Check sheet for the modelled part. Datum: model origin and axes. Units: mm. Face numbers are marked on the shaded views. A direction names the side the tool comes from. Round coordinates to 2 decimals unless told otherwise and drop trailing zeros. Loops run counter-clockwise (first coordinate to the right, second up) from the corner with the lowest first, then second, coordinate; pieces in that order, holes last. Notation, with made-up numbers: M -2,44.25 L 29,44.25 A12 ccw 29,55.25 Z; hole C -24.75,75 d2. An arc over 180 degrees is marked long. Write item = value, one per line. Start each with the question number.
(1) Set-up check for the marked faces 1 and 2: record each of +Z, -Z, +X, -X, +Y, -Y from which the full face is reachable in a straight line by a thin tool's end or side.
(2) Scan lines: L1, parallel to X at y = -7.25, z = 10.5; L2, parallel to X at y = -2.25, z = 14; L3, parallel to X at y = -1.5, z = -3.75. Record each from-to range of solid material in increasing order. Write a range as from..to.
(3) Cross-section at A-A on z = 2.75. Record the boundary of the cut face in (x, y), plus the area to 3 significant figures.
(4) Mould release check, pull along X, two halves, no side actions. Record for the marked faces 3, 4 and 5: pulls with the +X half, pulls with the -X half, needs draft (parallel to the pull), parting line crosses it, or undercut.
(5) Cross-section at C-C on y = -4.5. Record the boundary of the cut face in (x, z), plus the area to 3 significant figures.
(6) Cross-section at B-B on x = -12.5. Record the boundary of the cut face in (y, z).
(7) Cross-section at D-D on z = 11.5. Record the boundary of the cut face in (x, y), plus the area to 3 significant figures.
(8) Go/stop test with flat-tipped pins: P1, Ø2, axis at y = -10, z = 12, coming from the -X side; P2, Ø3, axis at y = -16, z = -1, coming from the +X side; P3, Ø1.5, axis at y = -8.5, z = 15, coming from the -X side. Record where each tip stops, or that it passes through.
from build123d import *

# Parameters (mm, degrees)
F0_R     = 1.5
F0_R_2   = 8.35
F1_DEPTH = 3
F2_DEPTH = 18
F3_R     = 3


with BuildPart() as f1:
    # F0 (on Front) → F1 (new body)
    with BuildSketch(Plane.XZ):
        Polygon((-48.303484, 19.342105), (-48.303484, 8.342105), (-37.303484, 19.342105), align=None)
        with Locations((-45.303484, 16.342105)):
            Circle(F0_R, mode=Mode.SUBTRACT)
        Polygon((-48.303484, 5.342105), (-48.303484, -5.657895), (-37.303484, -5.657895), align=None)
        with Locations((-45.303484, -2.657895)):
            Circle(F0_R, mode=Mode.SUBTRACT)
        Polygon((-48.303484, 5.342105), (-37.303484, -5.657895), (45.696516, -5.657895), (56.696516, 5.342105), (56.696516, 6.842105), (56.696516, 8.342105), (45.696516, 19.342105), (-37.303484, 19.342105), (-48.303484, 8.342105), (-48.303484, 6.842105), align=None)
        with Locations((-33.303484, 6.842105)):
            Circle(F0_R_2, mode=Mode.SUBTRACT)
        with Locations((-8.303484, 6.842105)):
            Circle(F0_R_2, mode=Mode.SUBTRACT)
        with Locations((16.696516, 6.842105)):
            Circle(F0_R_2, mode=Mode.SUBTRACT)
        with Locations((41.696516, 6.842105)):
            Circle(F0_R_2, mode=Mode.SUBTRACT)
        Polygon((45.696516, 19.342105), (56.696516, 8.342105), (56.696516, 19.342105), align=None)
        with Locations((53.696516, 16.342105)):
            Circle(F0_R, mode=Mode.SUBTRACT)
        Polygon((56.696516, 5.342105), (45.696516, -5.657895), (56.696516, -5.657895), align=None)
        with Locations((53.696516, -2.657895)):
            Circle(F0_R, mode=Mode.SUBTRACT)
    extrude(amount=F1_DEPTH)

    # F0 (on Front) → F2 (join)
    with BuildSketch(Plane.XZ):
        Polygon((-48.303484, 5.342105), (-37.303484, -5.657895), (45.696516, -5.657895), (56.696516, 5.342105), (56.696516, 6.842105), (56.696516, 8.342105), (45.696516, 19.342105), (-37.303484, 19.342105), (-48.303484, 8.342105), (-48.303484, 6.842105), align=None)
        with Locations((-33.303484, 6.842105)):
            Circle(F0_R_2, mode=Mode.SUBTRACT)
        with Locations((-8.303484, 6.842105)):
            Circle(F0_R_2, mode=Mode.SUBTRACT)
        with Locations((16.696516, 6.842105)):
            Circle(F0_R_2, mode=Mode.SUBTRACT)
        with Locations((41.696516, 6.842105)):
            Circle(F0_R_2, mode=Mode.SUBTRACT)
    extrude(amount=F2_DEPTH)

    # F3
    f3_edges = [f1.edges().sort_by_distance(p)[0] for p in [
        (-48.303484, -10.5, 8.342105),
        (-48.303484, -10.5, 5.342105),
        (56.696516, -10.5, 5.342105),
        (56.696516, -10.5, 8.342105),
    ]]
    fillet(f3_edges, radius=F3_R)


solid = f1.part
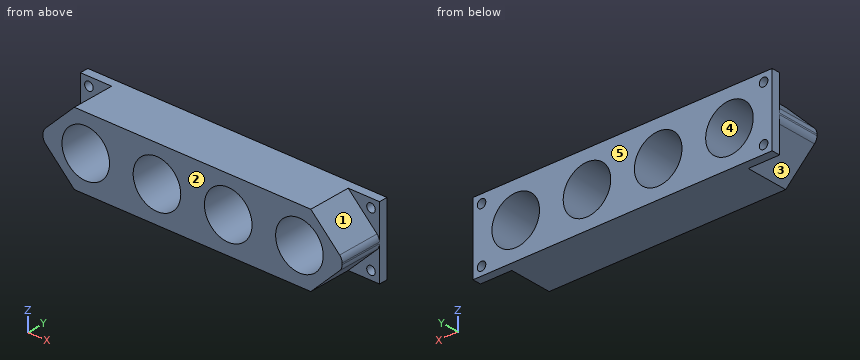
Result:
q1.face_1 = +Z, +X, -Y
q1.face_2 = +Z, -Z, +X, -X, -Y
q2.L1 = -46.15..-40.81, -25.8..-15.81, -0.8..9.19, 24.2..34.19, 49.2..54.54
q2.L2 = -48.3..-37.6, -29..-12.6, -4..12.4, 21..37.4, 46..56.7
q2.L3 = -48.3..-46.33, -44.28..52.67, 54.72..56.7
q3.outline = M -48.3,-3 L -45.71,-3 L -45.71,-18 L -40.58,-18 L -40.58,0 L -48.3,0 Z; M -26.02,-18 L -15.58,-18 L -15.58,0 L -26.02,0 Z; M -1.02,-18 L 9.42,-18 L 9.42,0 L -1.02,0 Z; M 23.98,-18 L 34.42,-18 L 34.42,0 L 23.98,0 Z; M 48.98,-18 L 54.1,-18 L 54.1,-3 L 56.7,-3 L 56.7,0 L 48.98,0 Z
q3.area = 764 mm^2
q4.face_3 = pulls with the -X half
q4.face_4 = undercut
q4.face_5 = needs draft
q5.outline = M -48.3,6.58 A3 ccw -47.42,4.46 L -37.3,-5.66 L 45.7,-5.66 L 55.82,4.46 A3 ccw 56.7,6.58 L 56.7,7.1 A3 ccw 55.82,9.22 L 45.7,19.34 L -37.3,19.34 L -47.42,9.22 A3 ccw -48.3,7.1 Z; hole C -33.3,6.84 d16.7; hole C -8.3,6.84 d16.7; hole C 16.7,6.84 d16.7; hole C 41.7,6.84 d16.7
q5.area = 1,510 mm^2
q6.outline = M -18,-5.66 L 0,-5.66 L 0,-0.38 L -18,-0.38 Z; M -18,14.06 L 0,14.06 L 0,19.34 L -18,19.34 Z
q7.outline = M -48.3,-3 L -45.15,-3 L -45.15,-18 L -40.23,-18 L -40.23,0 L -48.3,0 Z; M -26.37,-18 L -15.23,-18 L -15.23,0 L -26.37,0 Z; M -1.37,-18 L 9.77,-18 L 9.77,0 L -1.37,0 Z; M 23.63,-18 L 34.77,-18 L 34.77,0 L 23.63,0 Z; M 48.63,-18 L 53.54,-18 L 53.54,-3 L 56.7,-3 L 56.7,0 L 48.63,0 Z
q7.area = 797 mm^2
q8.P1 = -45.65
q8.P2 = 51.85
q8.P3 = -42.4
